from build123d import *

# Parameters (mm, degrees)
PAD_DEPTH = 1.5


with BuildPart() as part:
    # Sketch → Pad (new body)
    with BuildSketch(Plane(origin=(0, 0, 0), x_dir=(1, 0, 0), z_dir=(0, 0, -1))):
        with BuildLine():
            Line((9, 30), (9, 21.392622))
            ThreePointArc((-9, 21.392622), (0, -29), (9, 21.392622))
            Line((-9, 21.392622), (-9, 30))
            Line((-17, 30), (-9, 30))
            Line((-17, 63), (-17, 30))
            Line((-4.261222, 63), (-17, 63))
            Line((-4.261222, 63), (-4.261222, 65))
            Line((-4.261222, 65), (4.261222, 65))
            Line((4.261222, 65), (4.261222, 63))
            Line((17, 63), (4.261222, 63))
            Line((17, 30), (17, 63))
            Line((9, 30), (17, 30))
        make_face()
    extrude(amount=PAD_DEPTH)


solid = part.part
Could you check a few things on this model? Use its own coordinates, in mm. Coordinates: 2 decimals unless noted, no trailing zeros. Order: outer loops, then holes, each group sorted by start corner. A loop starts at its lowest first (then second) coordinate and runs counter-clockwise, first axis right, second up. Notation, with made-up numbers: (28, -20) - (32, -20) arc R18 cw to (32, -6) - close; hole circle Ø9 at (42, 12). An arc over 180 degrees is marked (long way). Answer in a Markdown table with one row per item. Add a question column.
(1) I need wall thicknesses on L1, parallel to X at y = -49, z = -1.05; L2, parallel to X at y = -29.5, z = -0.95; L3, parallel to Y at x = -10.5, z = -0.65. Which ranges of each line are inside material? Lowest first, please.
(2) If we section it at A-A, the plane z = -0.6: Please give me the cut outline in (x, y).
(3) If we section it at C-C, the plane x = -6: Please give me the cut outline in (y, z), then the cut area to 3 significant figures.
(4) Will this pin go through, and if not, where does the flat tip stop? pin 1 (0.8 mm diameter, centred on y = -27.5, z = -1, fed in from +X).
(5) If we section it at B-B, the plane y = -38.5: Please give me the cut outline in (x, z), then the cut area to 3 significant figures.
Results are:
| question | item | result |
|---|---|---|
| 1 | L1 | x = -17 to 17 |
| 1 | L2 | x = -9 to 9 |
| 1 | L3 | y = -63 to -30, -20.79 to 26.79 |
| 2 | outline | (-17, -63) - (-4.26, -63) - (-4.26, -65) - (4.26, -65) - (4.26, -63) - (17, -63) - (17, -30) - (9, -30) - (9, -21.39) arc R26 ccw (long way) to (-9, -21.39) - (-9, -30) - (-17, -30) - close |
| 3 | outline | (-63, -1.5) - (28.3, -1.5) - (28.3, 0) - (-63, 0) - close |
| 3 | area | 137 mm2 |
| 4 | pin 1 | stops at x = 9 |
| 5 | outline | (-17, -1.5) - (17, -1.5) - (17, 0) - (-17, 0) - close |
| 5 | area | 51.0 mm2 |
